from build123d import *

# Parameters (mm, degrees)
F1_DEPTH = 25.4
F3_DEPTH = 25.4


with BuildPart() as f1:
    # F0 (on Front) → F1 (new body)
    with BuildSketch(Plane.XZ):
        with BuildLine():
            Line((-28.17091, 55.533636), (-28.17091, -33.366363))
            Line((-28.17091, -33.366363), (13.392729, -33.366363))
            Line((13.392729, -33.366363), (13.392729, -7.042727))
            Line((13.392729, -7.042727), (32.789093, -7.042727))
            Line((32.789093, -7.042727), (32.789093, 55.533636))
            Line((32.789093, 55.533636), (17.549092, 55.533636))
            Line((17.549092, 55.533636), (17.549092, 34.837736))
            ThreePointArc((17.549092, 34.837736), (13.829348, 25.85748), (4.849092, 22.137736))
            Line((4.849092, 22.137736), (-0.230909, 22.137736))
            ThreePointArc((-0.230909, 22.137736), (-9.211165, 25.85748), (-12.930909, 34.837736))
            Line((-12.930909, 34.837736), (-12.930909, 55.533636))
            Line((-12.930909, 55.533636), (-28.17091, 55.533636))
        make_face()
    extrude(amount=F1_DEPTH)

    # F2 (on face) → F3 (join)
    with BuildSketch(Plane(origin=(0, 0, -33.366363), x_dir=(1, 0, 0), z_dir=(0, 0, -1))):
        with BuildLine():
            Line((-28.17091, 57.715932), (-28.17091, 0))
            Line((-28.17091, 0), (13.392729, 0))
            Line((13.392729, 0), (13.392729, 36.534619))
            Line((13.392729, 36.534619), (33.020001, 36.534619))
            Line((33.020001, 36.534619), (33.020001, 57.062088))
            ThreePointArc((33.020001, 57.062088), (2.727389, 85.731034), (-28.17091, 57.715932))
        make_face()
    extrude(amount=-F3_DEPTH)


solid = f1.part
Check sheet for the modelled part. Datum: model origin and axes. Units: mm. A direction names the side the tool comes from. Give positions to 0.01 mm unless a question says otherwise; leave off trailing zeros. Order: outer loops, then holes, each group sorted by start corner. A loop starts at its lowest first (then second) coordinate and runs counter-clockwise, first axis right, second up. Notation, with made-up numbers: M -35,63 L -6,63 A12 ccw -6,69 Z; hole C 67,83 d2. An arc over 180 degrees is marked long. Answer as CSV lines item,"result". Start each with the question number.
Item 1: Thickness scan on line 1 (Z direction, x = -24, y = -69); line 2 (X direction, y = -4.5, z = -24.5); line 3 (X direction, y = -7, z = 20). Record the ranges inside material, lowest first. Write a range as [from, to].
Item 2: Tool access check on faces 4 (the face through (-9.11, -12.52, 25.76)), 5 (the face through (2, -56, -7.966)), 6 (the face through (23, -36.535, -21)). Record the directions out of +Z, -Z, +X, -X, +Y, -Y that give a thin tool (end or side, any length) a straight path to the whole face; none if there is none.
Item 3: Cross-section at D-D on z = -22.5. Enter the section's corners in (x, y), plus the area to 3 significant figures.
Item 4: Cross-section at A-A on z = 36. Enter the section's corners in (x, y).
Item 5: Cross-section at C-C on y = -46.5. Enter the section's corners in (x, z).
Item 6: Mould release check, pull along X, two halves, no side actions. Record for faces 1 (the face through (-5, -43, -33.366)), 2 (the face through (-28.171, -23, 1)), 3 (the face through (13.93, -12.52, 25.96)): +X half, -X half, draft (parallel to the pull), parting line (faces both ways), or undercut.
Item 7: Gauge pin test, flat ends, axial feed: P1, Ø12, axis at x = 25.5, z = 30, coming from the -Y side; P2, Ø10.5, axis at y = -13, z = 47.5, coming from the +X side; P3, Ø8, axis at y = -20.5, z = -16, coming from the +X side. Record the tip position at first contact, or that the pin passes through.
Item 8: Cross-section at B-B on x = 27. Enter the section's corners in (y, z).
Established:
1,line 1,"z = [-33.37, -7.97]"
1,line 2,"x = [-28.17, 13.39]"
1,line 3,"x = [-28.17, 32.79]"
2,face 4,"+Z, +Y, -Y"
2,face 5,"+Z, +X, -X, -Y"
2,face 6,"+Z, -Z, +X, +Y"
3,outline,"M -28.17,-57.72 A30.69 ccw 33.02,-57.06 L 33.02,-36.53 L 13.39,-36.53 L 13.39,0 L -28.17,0 Z"
3,area,"4,130 mm^2"
4,outline,"M -28.17,-25.4 L -12.93,-25.4 L -12.93,0 L -28.17,0 Z; M 17.55,-25.4 L 32.79,-25.4 L 32.79,0 L 17.55,0 Z"
5,outline,"M -28.17,-33.37 L 33.02,-33.37 L 33.02,-7.97 L -28.17,-7.97 Z"
6,face 1,"draft"
6,face 2,"-X half"
6,face 3,"undercut"
7,P1,"stops at y = -25.4"
7,P2,"stops at x = 32.79"
7,P3,"stops at x = 13.39"
8,outline,"M -73.39,-33.37 L -36.53,-33.37 L -36.53,-7.97 L -73.39,-7.97 Z; M -25.4,-7.04 L 0,-7.04 L 0,55.53 L -25.4,55.53 Z"
